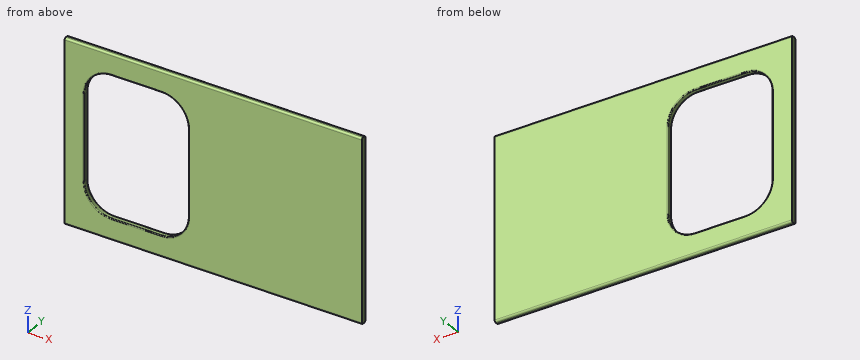
from build123d import *

# Parameters (mm, degrees)
SKETCH_1_W          = 165
SKETCH_1_H          = 100
EXTRUDE_1_DEPTH     = 3
SKETCH_2_W          = 57.969471509
SKETCH_2_H          = 76.82290634
CUT_EXTRUDE_1_DEPTH = 97.51554279
FILLET_1_R          = 15
FILLET_2_R          = 1
FILLET_3_R          = 0.5


with BuildPart() as part:
    # 草图1 → 凸台-拉伸1 (new body)
    with BuildSketch(Plane(origin=(0, 0, 0), x_dir=(1, 0, 0), z_dir=(0, 1, 0))):
        Rectangle(SKETCH_1_W, SKETCH_1_H)
    extrude(amount=EXTRUDE_1_DEPTH)

    # 草图2 → 切除-拉伸1 (cut, through all)
    with BuildSketch(Plane.XZ):
        with Locations((-42.70408642, 0)):
            Rectangle(SKETCH_2_W, SKETCH_2_H)
    extrude(amount=-CUT_EXTRUDE_1_DEPTH, mode=Mode.SUBTRACT)

    # 圆角1
    fillet_1_edges = [part.edges().sort_by_distance(p)[0] for p in [
        (-13.719350665, 1.5, 38.41145317),
        (-13.719350665, 1.5, -38.41145317),
        (-71.688822174, 1.5, -38.41145317),
        (-71.688822174, 1.5, 38.41145317),
    ]]
    fillet(fillet_1_edges, radius=FILLET_1_R)

    # 圆角2
    fillet_2_edges = [part.edges().sort_by_distance(p)[0] for p in [
        (0, 3, 50),
        (0, 0, 50),
        (0, 0, -50),
        (0, 3, -50),
    ]]
    fillet(fillet_2_edges, radius=FILLET_2_R)

    # 圆角3
    fillet_3_edges = [part.edges().sort_by_distance(p)[0] for p in [
        (-42.704086419, 0, -38.41145317),
        (-42.704086419, 3, -38.41145317),
        (-71.688822174, 0, 0),
        (-71.688822174, 3, 0),
        (-42.704086419, 0, 38.41145317),
        (-42.704086419, 3, 38.41145317),
        (-13.719350665, 0, 0),
        (-13.719350665, 3, 0),
        (-67.295423892, 0, -34.018054888),
        (-67.295423892, 3, -34.018054888),
        (-67.295423892, 0, 34.018054888),
        (-67.295423892, 3, 34.018054888),
        (-18.112748947, 0, -34.018054888),
        (-18.112748947, 3, -34.018054888),
        (-18.112748947, 0, 34.018054888),
        (-18.112748947, 3, 34.018054888),
    ]]
    fillet(fillet_3_edges, radius=FILLET_3_R)


solid = part.part
Work out the finished part from the listing and answer in its coordinate system (mm). Give positions to 0.01 mm unless a question says otherwise; leave off trailing zeros. Order: outer loops, then holes, each group sorted by start corner. A loop starts at its lowest first (then second) coordinate and runs counter-clockwise, first axis right, second up. Notation, with made-up numbers: (10.25, 11) -> (47.25, 11) arc R20 ccw to (47.25, 24) -> close; hole circle Ø8 at (55.25, 23.25). An arc over 180 degrees is marked (long way). Answer as a JSON object with one key per item and string values. Group by question number.
1. Section A-A on x = -42.5 is taken. Determine the outline of the cut face in (y, z), plus the area to 3 significant figures.
2. Section B-B on z = 16.5 is taken. Determine the outline of the cut face in (x, y), plus the area to 3 significant figures.
3. Consider line 1 along X through (y, z) = (2.6, -22); line 2 along Z through (x, y) = (-54, 2); line 3 along Z through (x, y) = (-18, 2.25). Determine where each line is inside the solid, lowest interval first. Write a range as [from, to].
Result sheet:
{
 "1": {"outline": "(0, -49) arc R1 ccw to (1, -50) -> (2, -50) arc R1 ccw to (3, -49) -> (3, -38.91) arc R0.5 ccw to (2.5, -38.41) -> (0.5, -38.41) arc R0.5 ccw to (0, -38.91) -> close; (0, 38.91) arc R0.5 ccw to (0.5, 38.41) -> (2.5, 38.41) arc R0.5 ccw to (3, 38.91) -> (3, 49) arc R1 ccw to (2, 50) -> (1, 50) arc R1 ccw to (0, 49) -> close", "area": "68.5 mm^2"},
 "2": {"outline": "(-82.5, 0) -> (-72.19, 0) arc R0.5 ccw to (-71.69, 0.5) -> (-71.69, 2.5) arc R0.5 ccw to (-72.19, 3) -> (-82.5, 3) -> close; (-13.72, 0.5) arc R0.5 ccw to (-13.22, 0) -> (82.5, 0) -> (82.5, 3) -> (-13.22, 3) arc R0.5 ccw to (-13.72, 2.5) -> close", "area": "321 mm^2"},
 "3": {"line 1": "x = [-82.5, -71.7], [-13.71, 82.5]", "line 2": "z = [-50, -38.41], [38.41, 50]", "line 3": "z = [-49.97, -33.9], [33.9, 49.97]"}
}
